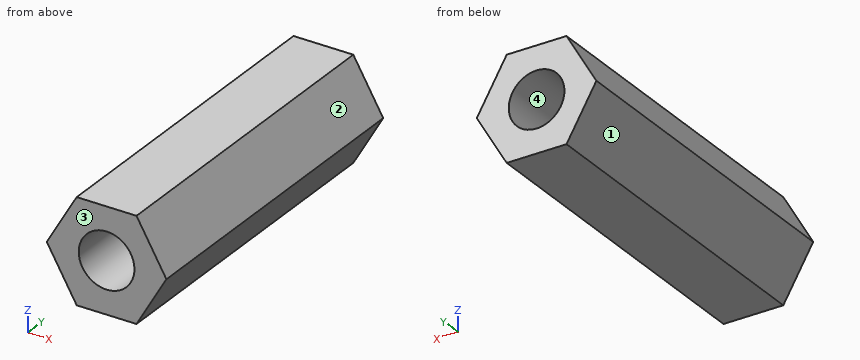
from build123d import *

# Parameters (mm, degrees)
BASE_DEPTH      = 15
HOLE_DEPTH      = 16.41470483
HOLE_DEPTH_BACK = 16.41470483
SKETCH2_R       = 1.25


with BuildPart() as part:
    # Sketch1 → base (new body)
    with BuildSketch(Plane(origin=(0, 0, 0), x_dir=(1, 0, 0), z_dir=(0, 1, 0))):
        Polygon((2.684678752, 0), (1.342339376, 2.325), (-1.342339376, 2.325), (-2.684678752, 0), (-1.342339376, -2.325), (1.342339376, -2.325), align=None)
    extrude(amount=BASE_DEPTH)

    # Sketch2 → hole (cut, two sides: drawn at the far end of the back side and taken through both)
    with BuildSketch(Plane(origin=(0, 15, 0), x_dir=(1, 0, 0), z_dir=(0, 1, 0)).offset(-HOLE_DEPTH_BACK)):
        with Locations(Location((0, 0, 0), (0, 0, 270))):
            Circle(SKETCH2_R)
    extrude(amount=HOLE_DEPTH + HOLE_DEPTH_BACK, mode=Mode.SUBTRACT)


solid = part.part
Here's how the part is built. I have some questions about the finished solid (model axes, mm). Face numbers are marked on the shaded views. Coordinates: 2 decimals unless noted, no trailing zeros. Write each loop counter-clockwise with the first axis right and the second up, starting at its lowest first coordinate (ties: lowest second). Pieces come first, ordered by that corner, then holes.
1) If I drill on line 1 (Z direction, x = 0, y = 8) (3 decimals); line 2 (X direction, y = 2, z = -0.45); line 3 (X direction, y = 5, z = 0.35), over which ranges is the centre line in solid material (lowest first)?
Filled in:
line 1: z = -2.325 to -1.25, 1.25 to 2.325
line 2: x = -2.42 to -1.17, 1.17 to 2.42
line 3: x = -2.48 to -1.2, 1.2 to 2.48
2) If we section it at A-A (x = 0.35): List the corners of the cut face in (y, z) for me (3 decimals).
Filled in:
outline: (0, -2.325) - (15, -2.325) - (15, -1.2) - (0, -1.2) - close; (0, 1.2) - (15, 1.2) - (15, 2.325) - (0, 2.325) - close
3) If we section it at D-D (z = -1.8): List the corners of the cut face in (x, y) for me, plus the area to 3 significant figures.
Filled in:
outline: (-1.65, 0) - (1.65, 0) - (1.65, 15) - (-1.65, 15) - close
area: 49.4 mm2
4) Thinking about a two-plate mould opening in X: for the marked faces 1, 2, 3 and 4, which applies, +X half, -X half, draft (parallel to the pull), parting line (faces both ways), or undercut?
Filled in:
face 1: -X half
face 2: +X half
face 3: draft
face 4: undercut
5) If we section it at C-C (y = 8): List the corners of the cut face in (x, z) for me (3 decimals).
Filled in:
outline: (-2.685, 0) - (-1.342, -2.325) - (1.342, -2.325) - (2.685, 0) - (1.342, 2.325) - (-1.342, 2.325) - close; hole circle Ø2.5 at (0, 0)
6) If we section it at B-B (z = 1): List the corners of the cut face in (x, y) for me, plus the area to 3 significant figures.
Filled in:
outline: (-2.11, 0) - (-0.75, 0) - (-0.75, 15) - (-2.11, 15) - close; (0.75, 0) - (2.11, 0) - (2.11, 15) - (0.75, 15) - close
area: 40.7 mm2
